Could you check a few things on this model? Use its own coordinates, in mm. Face numbers are marked on the shaded views. Coordinates: 2 decimals unless noted, no trailing zeros. Loops run counter-clockwise (first coordinate to the right, second up) from the corner with the lowest first, then second, coordinate; pieces in that order, holes last. Notation, with made-up numbers: (80.25, 25) -> (131.25, 25) arc R19 cw to (131.25, 49) -> close; hole circle Ø5 at (45, -40). An arc over 180 degrees is marked (long way). One line per question, with ' | ' between items. Start each with the question number.
(1) If we mould it in two halves opening along X, with no side actions, what happens to the marked faces 1, 2 and 3? For each: pulls with the +X half, pulls with the -X half, needs draft (parallel to the pull), parting line crosses it, or undercut.
(2) If I drill on line 1 along X through (y, z) = (19, 1); line 2 along Z through (x, y) = (8.5, 25); line 3 along X through (y, z) = (23, -2.5), over which ranges is the centre line in solid material (lowest first)?
(3) I'm going to push flat-ended pins straight in: pin 1 Ø14.5 at (x, z) = (4.15, -1.86) entering from +Y; pin 2 Ø11.5 at (x, z) = (4.15, -1.86) entering from -Y. Where does each tip first touch, or does it pass through?
(4) Suppose I cut it at A-A (y = 37.5). Please give me the cut outline in (x, z) (3 decimals), plus the area to 3 significant figures.
```python
from build123d import *

# Parameters (mm, degrees)
F0_W           = 101.6
F0_H           = 76.2
F1_DEPTH       = 50.8
F3_D           = 12.7
F3_CBORE_D     = 19.05
F3_CBORE_DEPTH = 6.35
F4_R           = 3.175
F5_SIZE        = 0.762


with BuildPart() as f1:
    # F0 (on Front) → F1 (new body)
    with BuildSketch(Plane.XZ):
        with Locations((4.1500981897, -1.8619502484)):
            Rectangle(F0_W, F0_H)
    extrude(amount=-F1_DEPTH)

    # F3 (through all)
    with Locations(Plane.XZ):
        with Locations((4.1500981897, -1.8619502484)):
            CounterBoreHole(F3_D / 2, F3_CBORE_D / 2, F3_CBORE_DEPTH)

    # F4
    f4_edges = [f1.edges().sort_by_distance(p)[0] for p in [
        (54.950098, 25.4, 36.23805),
        (-46.649902, 25.4, 36.23805),
        (54.950098, 25.4, -39.96195),
        (-46.649902, 25.4, -39.96195),
    ]]
    fillet(f4_edges, radius=F4_R)

    # F5
    f5_edges = [f1.edges().sort_by_distance(p)[0] for p in [
        (4.150098, 0, -39.96195),
        (-45.719966, 0, -39.032014),
        (54.020162, 0, -39.032014),
        (-46.649902, 0, -1.86195),
        (54.950098, 0, -1.86195),
        (-45.719966, 0, 35.308114),
        (54.020162, 0, 35.308114),
        (4.150098, 0, 36.23805),
        (-5.374902, 0, -1.86195),
    ]]
    chamfer(f5_edges, length=F5_SIZE)


solid = f1.part
```
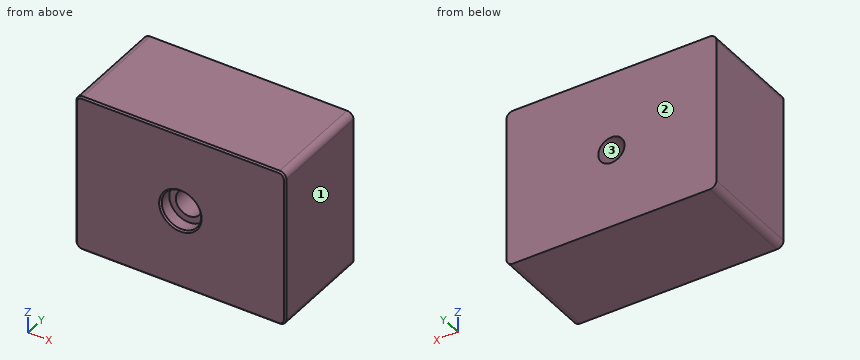
Checks:
1) face 1: pulls with the +X half | face 2: needs draft | face 3: undercut
2) line 1: x = -46.65 to -1.52, 9.82 to 54.95 | line 2: z = -39.96 to -6.49, 2.76 to 36.24 | line 3: x = -46.65 to -2.17, 10.47 to 54.95
3) pin 1: stops at y = 50.8 | pin 2: passes through
4) outline: (-46.65, -36.787) arc R3.175 ccw to (-43.475, -39.962) -> (51.775, -39.962) arc R3.175 ccw to (54.95, -36.787) -> (54.95, 33.063) arc R3.175 ccw to (51.775, 36.238) -> (-43.475, 36.238) arc R3.175 ccw to (-46.65, 33.063) -> close; hole circle Ø12.7 at (4.15, -1.862) | area: 7,610 mm^2
